```python
from build123d import *

# Parameters (mm, degrees)
BOSS_EXTRUDE1_DEPTH = 5.08
SKETCH2_W           = 5.08
SKETCH2_H           = 5.08
CUT_EXTRUDE1_DEPTH  = 5.08
CUT_EXTRUDE2_DEPTH  = 5.08


with BuildPart() as part:
    # Sketch1 → Boss-Extrude1 (new body)
    with BuildSketch(Plane(origin=(0, 0, 0), x_dir=(1, 0, 0), z_dir=(0, 1, 0))):
        Polygon((0, -45.356701101), (43.13678614, -14.015991449), (26.66, 36.694342), (-26.66, 36.694342), (-43.13678614, -14.015991449), align=None)
    extrude(amount=BOSS_EXTRUDE1_DEPTH)

    # Sketch2 → Cut-Extrude1 (cut)
    with BuildSketch(Plane(origin=(0, 5.08, 0), x_dir=(1, 0, 0), z_dir=(0, 1, 0))):
        with Locations((-17.78, 34.154342)):
            Rectangle(SKETCH2_W, SKETCH2_H)
        with Locations((7.62, 34.154342)):
            Rectangle(SKETCH2_W, SKETCH2_H)
        with Locations((17.78, 34.154342)):
            Rectangle(SKETCH2_W, SKETCH2_H)
        with Locations((-7.62, 34.154342)):
            Rectangle(SKETCH2_W, SKETCH2_H)
        Polygon((28.619167744, 30.664643686), (23.787800642, 29.094837355), (25.357606973, 24.263470252), (30.188974076, 25.833276584), align=None)
        Polygon((36.468199401, 6.507808173), (38.038005733, 1.67644107), (33.20663863, 0.106634738), (31.636832299, 4.938001841), align=None)
        Polygon((39.607812064, -3.154926033), (41.177618396, -7.986293136), (36.346251293, -9.556099467), (34.776444962, -4.724732364), align=None)
        Polygon((31.758780407, 21.001909481), (26.927413304, 19.432103149), (28.497219636, 14.600736047), (33.328586739, 16.170542378), align=None)
        Polygon((38.007618396, -17.742549949), (35.021669314, -13.632743617), (30.911862983, -16.618692699), (33.897812064, -20.72849903), align=None)
        Polygon((17.458586739, -32.672295357), (13.348780407, -35.658244439), (10.362831326, -31.548438107), (14.472637657, -28.562489025), align=None)
        Polygon((9.238974076, -38.64419352), (5.129167744, -41.630142602), (2.143218663, -37.52033627), (6.253024994, -34.534387189), align=None)
        Polygon((29.788005733, -23.714448112), (26.802056651, -19.60464178), (22.69225032, -22.590590862), (25.678199401, -26.700397194), align=None)
        Polygon((-5.129167744, -41.630142602), (-2.143218663, -37.52033627), (-6.253024994, -34.534387189), (-9.238974076, -38.64419352), align=None)
        Polygon((-25.678199401, -26.700397194), (-29.788005733, -23.714448112), (-26.802056651, -19.60464178), (-22.69225032, -22.590590862), align=None)
        Polygon((-33.897812064, -20.72849903), (-38.007618396, -17.742549949), (-35.021669314, -13.632743617), (-30.911862983, -16.618692699), align=None)
        Polygon((-13.348780407, -35.658244439), (-10.362831326, -31.548438107), (-14.472637657, -28.562489025), (-17.458586739, -32.672295357), align=None)
        Polygon((-41.177618396, -7.986293136), (-36.346251293, -9.556099467), (-34.776444962, -4.724732364), (-39.607812064, -3.154926033), align=None)
        Polygon((-33.328586739, 16.170542378), (-31.758780407, 21.001909481), (-26.927413304, 19.432103149), (-28.497219636, 14.600736047), align=None)
        Polygon((-30.188974076, 25.833276584), (-28.619167744, 30.664643686), (-23.787800642, 29.094837355), (-25.357606973, 24.263470252), align=None)
        Polygon((-38.038005733, 1.67644107), (-33.20663863, 0.106634738), (-31.636832299, 4.938001841), (-36.468199401, 6.507808173), align=None)
    extrude(amount=-CUT_EXTRUDE1_DEPTH, mode=Mode.SUBTRACT)

    # Sketch3 → Cut-Extrude2 (cut)
    with BuildSketch(Plane(origin=(0, 5.08, 0), x_dir=(1, 0, 0), z_dir=(0, 1, 0))):
        Polygon((0, 7.62), (2.54, 7.62), (2.54, 2.54), (7.62, 2.54), (7.62, 0), (7.62, -2.54), (2.54, -2.54), (2.54, -7.62), (0, -7.62), (-2.54, -7.62), (-2.54, -2.54), (-7.62, -2.54), (-7.62, 0), (-7.62, 2.54), (-2.54, 2.54), (-2.54, 7.62), align=None)
    extrude(amount=-CUT_EXTRUDE2_DEPTH, mode=Mode.SUBTRACT)


solid = part.part
```
The listing builds one solid part. Answer for the finished solid, in the listing's coordinates (mm). A direction names the side the tool comes from. Give positions to 0.01 mm unless a question says otherwise; leave off trailing zeros. Write each loop counter-clockwise with the first axis right and the second up, starting at its lowest first coordinate (ties: lowest second). Pieces come first, ordered by that corner, then holes. Notation, with made-up numbers: (39.25, 67.5) - (63.25, 67.5) arc R20 ccw to (63.25, 92.5) - close; hole circle Ø6 at (23, 27). An arc over 180 degrees is marked (long way). Use one line per item in the form item = value. Start each with the question number.
1) The mould has two halves that part along X. Classify faces 1 (the face through (11.27, 2.5, 37.17)), 2 (the face through (20.32, 3, -34)), 3 (the face through (-30.963, 2.504, -23.451)): pulls with the +X half, pulls with the -X half, needs draft (parallel to the pull), parting line crosses it, or undercut.
2) Find section A-A on z = 15. Determine the outline of the cut face in (x, y).
3) Consider line 1 along Z through (x, y) = (0, 3.75); line 2 along X through (y, z) = (3, 30); line 3 along Z through (x, y) = (-25.5, 0.95). Determine where each line is inside the solid, lowest interval first. Write a range as from..to.
4) A tool of negligible diameter and unlimited length cuts with its end or side. For faces 4 (the face through (7.725, 2.576, 36.561)), 5 (the face through (-8, 3, -31.614)), 6 (the face through (-2.54, 3, -5)), from which of +Z, -Z, +X, -X, +Y, -Y can it reach the whole face along a straight path? Write none if from no direction.
5) Flat-ended cylindrical pins translate along their axes: pin 1 Ø2.5 at (x, y) = (-8, 2) entering from -Z; pin 2 Ø1.5 at (y, z) = (4, 31.5) entering from -X; pin 3 Ø10 at (x, z) = (-1, -26.5) entering from -Y; pin 4 Ø2.5 at (y, z) = (3.5, 1) entering from -X. Find the tip coordinate at first contact, or state that the pin passes through.
6) Find section B-B on z = -9. Determine the outline of the cut face in (x, y).
Geometry results:
q1.face_1 = pulls with the +X half
q1.face_2 = undercut
q1.face_3 = pulls with the -X half
q2.outline = (-41.78, 0) - (-36.02, 0) - (-36.02, 5.08) - (-41.78, 5.08) - close; (-33.14, 0) - (33.14, 0) - (33.14, 5.08) - (-33.14, 5.08) - close; (36.02, 0) - (41.78, 0) - (41.78, 5.08) - (36.02, 5.08) - close
q3.line_1 = -36.69..-7.62, 7.62..45.36
q3.line_2 = -21.14..-15.52, -12.49..12.49, 15.52..21.14
q3.line_3 = -36.69..-29.65, -24.31..20.55, 26.46..26.83
q4.face_4 = +Z, +Y, -Y
q4.face_5 = -Z, +Y, -Y
q4.face_6 = +Y, -Y
q5.pin_1 = -31.61
q5.pin_2 = -20.1
q5.pin_3 = 0
q5.pin_4 = -39.31
q6.outline = (-35.66, 0) - (35.66, 0) - (35.66, 5.08) - (-35.66, 5.08) - close
